from build123d import *

# Parameters (mm, degrees)
ESBO_O1_W                = 9.53
ESBO_O1_H                = 10.03
RESSALTO_EXTRUS_O1_DEPTH = 2.415
CORTE_EXTRUS_O1_REACH    = 6.83
ESBO_O2_W                = 7.93
ESBO_O2_H                = 1
CORTE_EXTRUS_O2_DEPTH    = 0.38
ESBO_O4_R                = 1.095
RESSALTO_EXTRUS_O2_DEPTH = 1.52
CORTE_EXTRUS_O3_DEPTH    = 0.5
ESBO_O6_R                = 0.255
RESSALTO_EXTRUS_O3_DEPTH = 2.98


with BuildPart() as part:
    # Esboço1 → Ressalto-extrusão1 (new body, symmetric)
    with BuildSketch(Plane(origin=(0, 0, 0), x_dir=(1, 0, 0), z_dir=(0, 1, 0))):
        with Locations((0, -5.015)):
            Rectangle(ESBO_O1_W, ESBO_O1_H)
    extrude(amount=RESSALTO_EXTRUS_O1_DEPTH, both=True)

    # Esboço2 → Corte-extrusão1 (cut, up to next)
    with BuildSketch(Plane(origin=(0, -2.415, 0), x_dir=(-1, 0, 0), z_dir=(0, -1, 0)), mode=Mode.PRIVATE) as corte_extrus_o1_sk1:
        with Locations((0, 0.12)):
            Rectangle(ESBO_O2_W, ESBO_O2_H)
    corte_extrus_o1_tool1 = extrude(corte_extrus_o1_sk1.sketch, amount=-CORTE_EXTRUS_O1_REACH, mode=Mode.PRIVATE) & part.part
    add(corte_extrus_o1_tool1.solids().sort_by_distance((0, -2.415, -0.12))[0], mode=Mode.SUBTRACT)

    # Esboço3 → Corte-extrusão2 (cut)
    with BuildSketch(Plane(origin=(0, 2.415, 0), x_dir=(1, 0, 0), z_dir=(0, 1, 0))):
        Polygon((3.965, -0.38), (-3.965, -0.38), (-3.965, -1), (-4.765, -1), (-4.765, -9.03), (-3.965, -9.03), (-3.965, -10.03), (3.965, -10.03), (3.965, -9.03), (4.765, -9.03), (4.765, -1), (3.965, -1), align=None)
    extrude(amount=-CORTE_EXTRUS_O2_DEPTH, mode=Mode.SUBTRACT)

    # Esboço4 → Ressalto-extrusão2 (add)
    with BuildSketch(Plane.XY.offset(10.03)):
        with Locations((3.495, -1.145)):
            Circle(ESBO_O4_R)
    extrude(amount=RESSALTO_EXTRUS_O2_DEPTH)

    # Esboço5 → Corte-extrusão3 (cut)
    with BuildSketch(Plane.XY.offset(11.55)):
        with BuildLine():
            Line((2.917944817, -0.214391427), (4.425608573, -1.722055183))
            ThreePointArc((4.425608573, -1.722055183), (4.269281925, -1.919281925), (4.072055183, -2.075608573))
            Line((4.072055183, -2.075608573), (2.564391427, -0.567944817))
            ThreePointArc((2.564391427, -0.567944817), (2.720718075, -0.370718075), (2.917944817, -0.214391427))
        make_face()
    extrude(amount=-CORTE_EXTRUS_O3_DEPTH, mode=Mode.SUBTRACT)

    # Esboço6 → Ressalto-extrusão3 (add)
    with BuildSketch(Plane(origin=(0, 0, 0.38), x_dir=(-1, 0, 0), z_dir=(0, 0, -1))):
        with Locations((0, 0.005)):
            Circle(ESBO_O6_R)
        with Locations((-2.54, 0.005)):
            Circle(ESBO_O6_R)
        with Locations((2.54, 0.005)):
            Circle(ESBO_O6_R)
    extrude(amount=RESSALTO_EXTRUS_O3_DEPTH)


solid = part.part
The model under review builds one solid part; all positions refer to its coordinate system, in mm. A direction names the side the tool comes from. Round coordinates to 2 decimals unless told otherwise and drop trailing zeros. Order: outer loops, then holes, each group sorted by start corner. A loop starts at its lowest first (then second) coordinate and runs counter-clockwise, first axis right, second up. Notation, with made-up numbers: (15, 40.25) -> (68, 40.25) arc R27 ccw to (68, 68.25) -> close; hole circle Ø4 at (26.25, -33). An arc over 180 degrees is marked (long way). Write item = value, one per line. Start each with the question number.
Item 1: Consider section B-B on y = 1.55. Write out the cut boundary in (x, z) (3 decimals).
Item 2: Mouldability with a two-part tool opening along Y and no side actions: class faces 5 (the face through (0, -2.415, 5)), 6 (the face through (3.661, -0.958, 11.304)), 7 (the face through (4, -1, 11.55)) as released by +Y, released by -Y, zero draft, split by the parting line, or undercut.
Item 3: Consider section A-A on x = -2.54. Write out the cut boundary in (y, z) (3 decimals), plus the area to 3 significant figures.
Item 4: Clearance check with flat-ended pins moving along their axes: pin 1 Ø1 at (x, z) = (3.5, 8) entering from +Y (3 decimals); pin 2 Ø1 at (x, y) = (0.5, 0) entering from +Z. State where each tip first meets the part, or that it passes through.
Item 5: For faces 1 (the face through (-3.965, 0.6, 0.2)), 2 (the face through (3, -1.6, 11.55)), 3 (the face through (3.57, -1.14, 11.05)), 4 (the face through (0, -1, 0.38)), list the 3-axis set-ups (+Z, -Z, +X, -X, +Y, -Y) from which the entire face can be reached by the end or side of a thin tool; tool diameter is ignored.
Item 6: For line 1 along X through (y, z) = (0.2, -1); line 2 along Z through (x, y) = (-3, -1.3); line 3 along Y through (x, z) = (3, 5.75) (3 decimals), list the stretches that pass through material, from the lowest coordinate up.
Item 7: Consider section C-C on z = 4.75. Write out the cut boundary in (x, y) (3 decimals), plus the area to 3 significant figures.
Item 8: Consider section D-D on x = 3.25. Write out the cut boundary in (y, z) (3 decimals).
Conclusion:
q1.outline = (-4.765, 0) -> (-3.965, 0) -> (-3.965, 0.38) -> (3.965, 0.38) -> (3.965, 0) -> (4.765, 0) -> (4.765, 10.03) -> (-4.765, 10.03) -> close
q2.face_5 = released by -Y
q2.face_6 = undercut
q2.face_7 = zero draft
q3.outline = (-2.415, 0.38) -> (-0.25, 0.38) -> (-0.25, -2.6) -> (0.26, -2.6) -> (0.26, 0.38) -> (2.035, 0.38) -> (2.035, 10.03) -> (-2.415, 10.03) -> close
q3.area = 44.5 mm2
q4.pin_1 = 2.035
q4.pin_2 = 10.03
q5.face_1 = -Z, +Y
q5.face_2 = +Z, +X, -X, +Y, -Y
q5.face_3 = +Z
q5.face_4 = -Z
q6.line_1 = -2.7 to -2.38, -0.16 to 0.16, 2.38 to 2.7
q6.line_2 = 0.38 to 10.03
q6.line_3 = -2.415 to 2.035
q7.outline = (-4.765, -2.415) -> (4.765, -2.415) -> (4.765, 2.035) -> (-4.765, 2.035) -> close
q7.area = 42.4 mm2
q8.outline = (-2.415, 0.38) -> (2.035, 0.38) -> (2.035, 10.03) -> (-0.078, 10.03) -> (-0.078, 11.55) -> (-0.546, 11.55) -> (-0.546, 11.05) -> (-1.254, 11.05) -> (-1.254, 11.55) -> (-2.212, 11.55) -> (-2.212, 10.03) -> (-2.415, 10.03) -> close
